```python
from build123d import *

# Parameters (mm, degrees)
SKETCH1_R           = 2.8
BOSS_EXTRUDE1_DEPTH = 67
SKETCH2_R           = 3.25
CUT_EXTRUDE1_DEPTH  = 100
BOSS_EXTRUDE2_DEPTH = 5.5
CUT_EXTRUDE2_DEPTH  = 1.6
FILLET1_R           = 1.6
FILLET2_R           = 5


with BuildPart() as part:
    # Sketch1 → Boss-Extrude1 (new body)
    with BuildSketch(Plane.XY):
        with BuildLine():
            Line((16.248076809, -3.5), (40, -3.5))
            Line((40, -3.5), (40, -7.5))
            Line((40, -7.5), (0, -7.5))
            ThreePointArc((0, -7.5), (-6.210590034, 4.204589329), (6.96346149, 2.785714286))
            ThreePointArc((6.96346149, 2.785714286), (10.641957703, -1.780786712), (16.248076809, -3.5))
        make_face()
        Circle(SKETCH1_R, mode=Mode.SUBTRACT)
    extrude(amount=BOSS_EXTRUDE1_DEPTH)

    # Sketch2 → Cut-Extrude1 (cut)
    with BuildSketch(Plane(origin=(0, -3.5, 0), x_dir=(1, 0, 0), z_dir=(0, 1, 0))):
        with Locations(Location((22.248076809, -33.5, 0), (0, 0, 270))):
            Circle(SKETCH2_R)
    extrude(amount=-CUT_EXTRUDE1_DEPTH, mode=Mode.SUBTRACT)

    # Sketch3 → Boss-Extrude2 (add, symmetric)
    with BuildSketch(Plane.XY.offset(33.5)):
        with BuildLine():
            Line((30.94, -3.5), (40, -3.5))
            Line((40, -3.5), (40, 2.5))
            ThreePointArc((40, 2.5), (35.47, -2.03), (30.94, 2.5))
            Line((30.94, 2.5), (30.94, -3.5))
        make_face()
        with BuildLine():
            ThreePointArc((30.94, 2.5), (35.47, -2.03), (40, 2.5))
            Line((40, 2.5), (37.248, 2.5))
            ThreePointArc((37.248, 2.5), (35.47, 0.722), (33.692, 2.5))
            Line((33.692, 2.5), (30.94, 2.5))
        make_face()
        with BuildLine():
            Line((37.248, 2.5), (40, 2.5))
            ThreePointArc((40, 2.5), (35.47, 7.03), (30.94, 2.5))
            Line((30.94, 2.5), (33.692, 2.5))
            ThreePointArc((33.692, 2.5), (35.47, 4.278), (37.248, 2.5))
        make_face()
    extrude(amount=BOSS_EXTRUDE2_DEPTH, both=True)

    # Sketch3_3 → Cut-Extrude2 (cut, symmetric)
    with BuildSketch(Plane.XY.offset(33.5)):
        with BuildLine():
            Line((30.94, -3.5), (40, -3.5))
            Line((40, -3.5), (40, 2.5))
            ThreePointArc((40, 2.5), (35.47, -2.03), (30.94, 2.5))
            Line((30.94, 2.5), (30.94, -3.5))
        make_face()
        with BuildLine():
            ThreePointArc((30.94, 2.5), (35.47, -2.03), (40, 2.5))
            Line((40, 2.5), (37.248, 2.5))
            ThreePointArc((37.248, 2.5), (35.47, 0.722), (33.692, 2.5))
            Line((33.692, 2.5), (30.94, 2.5))
        make_face()
        with BuildLine():
            Line((37.248, 2.5), (40, 2.5))
            ThreePointArc((40, 2.5), (35.47, 7.03), (30.94, 2.5))
            Line((30.94, 2.5), (33.692, 2.5))
            ThreePointArc((33.692, 2.5), (35.47, 4.278), (37.248, 2.5))
        make_face()
    extrude(amount=CUT_EXTRUDE2_DEPTH, both=True, mode=Mode.SUBTRACT)

    # Fillet1
    fillet1_edges = [part.edges().sort_by_distance(p)[0] for p in [
        (35.47, -3.5, 39),
        (30.94, -3.5, 37.05),
        (35.47, -3.5, 28),
        (30.94, -3.5, 29.95),
    ]]
    fillet(fillet1_edges, radius=FILLET1_R)

    # Fillet2
    fillet2_edges = [part.edges().sort_by_distance(p)[0] for p in [
        (40, -5.5, 67),
        (40, -5.5, 0),
    ]]
    fillet(fillet2_edges, radius=FILLET2_R)


solid = part.part
```
Build history of the part. All positions in model axes, mm. A direction names the side the tool comes from. Round coordinates to 2 decimals unless told otherwise and drop trailing zeros. Order: outer loops, then holes, each group sorted by start corner. A loop starts at its lowest first (then second) coordinate and runs counter-clockwise, first axis right, second up. Notation, with made-up numbers: (3, -23) - (42, -23) arc R21 cw to (42, -15) - close; hole circle Ø6 at (-33.5, 72). An arc over 180 degrees is marked (long way). Use a Markdown table: item, result.
1) Wall check: L1, parallel to Z at x = 33, y = -1; L2, parallel to Y at x = 22, z = 24.5; L3, parallel to X at y = -2.25, z = 6.5. Give the ranges that are in metal, low to high.
Recorded:
| item | result |
|---|---|
| L1 | z = 28 to 31.9, 35.1 to 39 |
| L2 | y = -7.5 to -3.5 |
| L3 | x = -7.15 to -1.67, 1.67 to 11.41 |
2) Saw through at A-A on z = 33.5. Write the cut outline in (x, y).
Recorded:
| item | result |
|---|---|
| outline | (0, -7.5) - (19, -7.5) - (19, -3.5) - (16.25, -3.5) arc R10 cw to (6.96, 2.79) arc R7.5 ccw (long way) to start; (25.5, -7.5) - (40, -7.5) - (40, -3.5) - (25.5, -3.5) - close; hole circle Ø5.6 at (0, 0) |
3) Pull direction X, two halves, no side cores. Call faces 5 (the face through (30.94, 0, 30)), 6 (the face through (38, -6, 66)), 7 (the face through (34.74, -3.04, 27.52)): pulls with the +X half, pulls with the -X half, needs draft (parallel to the pull), parting line crosses it, or undercut.
Recorded:
| item | result |
|---|---|
| face 5 | undercut |
| face 6 | pulls with the +X half |
| face 7 | needs draft |
4) Tool access for faces 1 (the face through (34.74, -3.04, 39.48)), 2 (the face through (36.4, 0.6, 28)), 3 (the face through (30.5, -3, 29.8)), 4 (the face through (34.6, 0.7, 35.1)): list every direction of +Z, -Z, +X, -X, +Y, -Y with a clear straight run to the whole face (end or side of a thin tool).
Recorded:
| item | result |
|---|---|
| face 1 | +Z, +X, +Y |
| face 2 | -Z, +X, +Y |
| face 3 | +Z, -Z, +Y |
| face 4 | +X, +Y |
5) Saw through at B-B on y = -0.75. Write the cut outline in (x, z), and give its area (3 significant figures).
Recorded:
| item | result |
|---|---|
| outline | (-7.46, 0) - (-2.7, 0) - (-2.7, 67) - (-7.46, 67) - close; (2.7, 0) - (9.36, 0) - (9.36, 67) - (2.7, 67) - close; (30.94, 28) - (40, 28) - (40, 31.9) - (30.94, 31.9) - close; (30.94, 35.1) - (40, 35.1) - (40, 39) - (30.94, 39) - close |
| area | 836 mm² |
6) Flat gauge pins, fed straight in: pin 1 Ø3 at (y, z) = (2.5, 57) entering from -X; pin 2 Ø2 at (y, z) = (-5, 48.5) entering from -X; pin 3 Ø3 at (x, y) = (34.5, 0.5) entering from +Z. Where does each tip first touch, or does it go through?
Recorded:
| item | result |
|---|---|
| pin 1 | stops at x = -7.43 |
| pin 2 | stops at x = -6.34 |
| pin 3 | stops at z = 39 |
7) Saw through at C-C on z = 13.5. Write the cut outline in (x, y), and give its area (3 significant figures).
Recorded:
| item | result |
|---|---|
| outline | (0, -7.5) - (40, -7.5) - (40, -3.5) - (16.25, -3.5) arc R10 cw to (6.96, 2.79) arc R7.5 ccw (long way) to start; hole circle Ø5.6 at (0, 0) |
| area | 307 mm² |
